Read the model definition and answer for the solid it produces. Units are mm, in the model's axes. Face numbers are marked on the shaded views. A direction names the side the tool comes from. Round coordinates to 2 decimals unless told otherwise and drop trailing zeros. Order: outer loops, then holes, each group sorted by start corner. A loop starts at its lowest first (then second) coordinate and runs counter-clockwise, first axis right, second up. Notation, with made-up numbers: (26.25, 41.5) - (39.25, 41.5) arc R20 ccw to (39.25, 49.5) - close; hole circle Ø11 at (67, 37). An arc over 180 degrees is marked (long way). Answer as a JSON object with one key per item and string values. Group by question number.
Q1. A cutting plane is placed at B-B on y = 6.5. Determine the outline of the cut face in (x, z), and give its area (4 significant figures).
Q2. A tool of negligible diameter and unlimited length cuts with its end or side. For the marked faces 4, 5, 6 and 7, from which of +Z, -Z, +X, -X, +Y, -Y can it reach the whole face along a straight path? Write none if from no direction.
Q3. The mould has two halves that part along Z. Classify the marked faces 1, 2 and 3: pulls with the +Z half, pulls with the -Z half, needs draft (parallel to the pull), parting line crosses it, or undercut.
Q4. A cutting plane is placed at D-D on y = 11.5. Determine the outline of the cut face in (x, z).
Q5. A cutting plane is placed at C-C on x = -29.25. Determine the outline of the cut face in (y, z), and give its area (3 significant figures).
Q6. Given pin 1 Ø2.5 at (x, y) = (-12, 4.5) entering from +Z; pin 2 Ø5 at (x, z) = (-22, 4) entering from -Y; pin 3 Ø0.9 at (x, y) = (-22, 11.5) entering from +Z, each flat-ended and moving along its own axis, determine where each tip first touches the part or whether it passes through.
Q7. Consider line 1 (Z direction, x = -8.75, y = 4.5); line 2 (Y direction, x = -22.5, z = 0); line 3 (Z direction, x = -21.25, y = 11.5). Determine where each line is inside the solid, lowest interval first.
Q8. A cutting plane is placed at A-A on z = 0.5. Determine the outline of the cut face in (x, y), and give its area (4 significant figures).
```python
from build123d import *

# Parameters (mm, degrees)
SKETCH1_W               = 30
SKETCH1_H               = 15
BOSS_EXTRUDE1_DEPTH     = 15
CUT_EXTRUDE1_DEPTH      = 1.55
CUT_EXTRUDE1_DEPTH_BACK = 1.55
SKETCH2_W               = 30
SKETCH2_H               = 8
CUT_EXTRUDE2_DEPTH      = 1.55
CUT_EXTRUDE2_DEPTH_BACK = 1.55
SKETCH4_W               = 30
SKETCH4_H               = 8
SKETCH5_W               = 8.45
SKETCH5_H               = 8.45
CUT_EXTRUDE3_DEPTH      = 35.431000961
FILLET1_R               = 3


with BuildPart() as part:
    # Sketch1 → Boss-Extrude1 (new body)
    with BuildSketch(Plane(origin=(0, 0, 0), x_dir=(1, 0, 0), z_dir=(0, 1, 0))):
        with Locations((-19.236111111, 0.277777778)):
            Rectangle(SKETCH1_W, SKETCH1_H)
    extrude(amount=BOSS_EXTRUDE1_DEPTH)

    # Sketch2 → Cut-Extrude1 (cut, two sides: drawn at the far end of the back side and taken through both)
    with BuildSketch(Plane(origin=(0, 0, -4.777777778), x_dir=(-1, 0, 0), z_dir=(0, 0, -1)).offset(-CUT_EXTRUDE1_DEPTH_BACK)):
        with Locations((19.236111111, 4)):
            Rectangle(SKETCH2_W, SKETCH2_H)
    extrude(amount=CUT_EXTRUDE1_DEPTH + CUT_EXTRUDE1_DEPTH_BACK, mode=Mode.SUBTRACT)

    # Sketch4 → Cut-Extrude2 (cut, two sides: drawn at the far end of the back side and taken through both)
    with BuildSketch(Plane(origin=(0, 12, 0), x_dir=(1, 0, 0), z_dir=(0, 1, 0)).offset(-CUT_EXTRUDE2_DEPTH_BACK)):
        with Locations((-19.236111111, -3.222222222)):
            Rectangle(SKETCH4_W, SKETCH4_H)
    extrude(amount=CUT_EXTRUDE2_DEPTH + CUT_EXTRUDE2_DEPTH_BACK, mode=Mode.SUBTRACT)

    # Sketch5 → Cut-Extrude3 (cut, through all)
    with BuildSketch(Plane.ZY.offset(34.236111111)):
        with Locations((2.997222222, 4.225)):
            Rectangle(SKETCH5_W, SKETCH5_H)
    extrude(amount=-CUT_EXTRUDE3_DEPTH, mode=Mode.SUBTRACT)

    # Fillet1
    # the kernel refuses this fillet: 3 mm, written as the material it takes off along each edge
    with BuildSketch(Plane(origin=(2.185288658, 15, 7.222222222), x_dir=(0, 0, -1), z_dir=(-1, 0, 0)), Plane(origin=(-40.657510881, 0, -7.777777778), x_dir=(0, 1, 0), z_dir=(1, 0, 0))) as fillet1_piece_1:
        with BuildLine():
            CenterArc((2.568559908, 3), FILLET1_R, 211.108922511, 58.891077489)
            Line((0, 1.45), (-0.051371198, 1.419))
            ThreePointArc((-0.051371198, 1.419), (-0.06, 0.725), (-0.06, 0))
            Line((-0.06, 0), (0, -0.06))
            Line((0, -0.06), (2.568559908, -0.06))
            Line((2.568559908, -0.06), (2.568559908, 0))
        make_face()
    extrude(amount=42.842799539, mode=Mode.SUBTRACT)
    with BuildSketch(Plane(origin=(-41.736111111, 15, -7.777777778), x_dir=(0, -1, 0), z_dir=(1, 0, 0))) as fillet1_piece_2:
        with BuildLine():
            CenterArc((FILLET1_R, -FILLET1_R), FILLET1_R, 90, 90)
            Line((0, -FILLET1_R), (-FILLET1_R * 0.02, -FILLET1_R))
            Line((-FILLET1_R * 0.02, -FILLET1_R), (-FILLET1_R * 0.02, FILLET1_R * 0.02))
            Line((-FILLET1_R * 0.02, FILLET1_R * 0.02), (FILLET1_R, FILLET1_R * 0.02))
            Line((FILLET1_R, FILLET1_R * 0.02), (FILLET1_R, 0))
        make_face()
    extrude(amount=45, mode=Mode.SUBTRACT)


solid = part.part
```
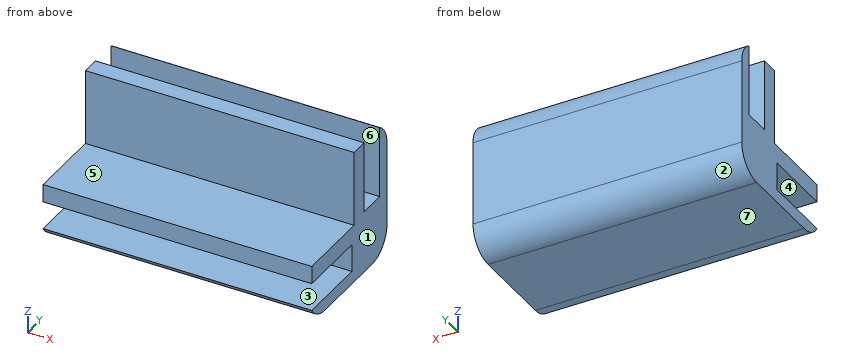
Result set:
{
 "1": {"outline": "(-34.24, -7.78) - (-4.24, -7.78) - (-4.24, -6.33) - (-34.24, -6.33) - close; (-34.24, -3.23) - (-4.24, -3.23) - (-4.24, -1.23) - (-34.24, -1.23) - close", "area": "103.5 mm²"},
 "2": {"face 4": "+X, -X, -Y", "face 5": "+Z, +X, -X, -Y", "face 6": "+Z, +X, -X", "face 7": "-Z, +X, -X, +Y, -Y"},
 "3": {"face 1": "needs draft", "face 2": "pulls with the -Z half", "face 3": "undercut"},
 "4": {"outline": "(-34.24, -7.78) - (-4.24, -7.78) - (-4.24, -0.78) - (-34.24, -0.78) - close"},
 "5": {"outline": "(0, -6.33) arc R3 ccw to (2.57, -7.78) - (12, -7.78) arc R3 ccw to (15, -4.78) - (15, 4.65) arc R3 ccw to (13.55, 7.22) - (13.55, -0.78) - (10.45, -0.78) - (10.45, 7.22) - (8.45, 7.22) - (8.45, -1.23) - (0, -1.23) - (0, -3.23) - (8, -3.23) - (8, -6.33) - close", "area": "99.9 mm²"},
 "6": {"pin 1": "stops at z = -1.23", "pin 2": "stops at y = 8.45", "pin 3": "stops at z = -0.78"},
 "7": {"line 1": "z = -7.78 to -6.33, -3.23 to -1.23", "line 2": "y = 8.45 to 10.45, 13.55 to 15", "line 3": "z = -7.78 to -0.78"},
 "8": {"outline": "(-34.24, 8.45) - (-4.24, 8.45) - (-4.24, 10.45) - (-34.24, 10.45) - close; (-34.24, 13.55) - (-4.24, 13.55) - (-4.24, 15) - (-34.24, 15) - close", "area": "103.5 mm²"}
}
